from build123d import *

# Parameters (mm, degrees)
F0_R     = 10
F1_DEPTH = 5


with BuildPart() as f1:
    # F0 (on Front) → F1 (new body)
    with BuildSketch(Plane.XZ):
        Circle(F0_R)
        with BuildLine():
            ThreePointArc((-3.708099, -1.5), (-2.828427, -2.828427), (-1.5, -3.708099))
            Line((-1.5, -3.708099), (-1.5, -7.348469))
            ThreePointArc((-1.5, -7.348469), (-5.303301, -5.303301), (-7.348469, -1.5))
            Line((-7.348469, -1.5), (-3.708099, -1.5))
        make_face(mode=Mode.SUBTRACT)
        with BuildLine():
            Line((3.708099, -1.5), (7.348469, -1.5))
            ThreePointArc((7.348469, -1.5), (5.303301, -5.303301), (1.5, -7.348469))
            Line((1.5, -7.348469), (1.5, -3.708099))
            ThreePointArc((1.5, -3.708099), (2.828427, -2.828427), (3.708099, -1.5))
        make_face(mode=Mode.SUBTRACT)
        with BuildLine():
            Line((-1.5, 7.348469), (-1.5, 3.708099))
            ThreePointArc((-1.5, 3.708099), (-2.828427, 2.828427), (-3.708099, 1.5))
            Line((-3.708099, 1.5), (-7.348469, 1.5))
            ThreePointArc((-7.348469, 1.5), (-5.303301, 5.303301), (-1.5, 7.348469))
        make_face(mode=Mode.SUBTRACT)
        with BuildLine():
            Line((1.5, 3.708099), (1.5, 7.348469))
            ThreePointArc((1.5, 7.348469), (5.303301, 5.303301), (7.348469, 1.5))
            Line((7.348469, 1.5), (3.708099, 1.5))
            ThreePointArc((3.708099, 1.5), (2.828427, 2.828427), (1.5, 3.708099))
        make_face(mode=Mode.SUBTRACT)
    extrude(amount=F1_DEPTH)


solid = f1.part
Input: part model. Units: mm. Frame: model coordinates. A direction names the side the tool comes from. Round coordinates to 2 decimals unless told otherwise and drop trailing zeros. Order: outer loops, then holes, each group sorted by start corner. A loop starts at its lowest first (then second) coordinate and runs counter-clockwise, first axis right, second up.
1. Set-up query: faces 4 (the face through (0, -5, 0)), 5 (the face through (-6, -2, -1.5)). Return all of +Z, -Z, +X, -X, +Y, -Y with unobstructed straight access to the full face (end or side cutting, diameter ignored); none if empty.
The answers:
face 4: +Z, -Z, +X, -X, -Y
face 5: +Y, -Y
2. Cut plane A-A, the plane y = -4.05. Output: boundary loops of the cut face in (x, z).
The answers:
outline: circle Ø20 at (0, 0); hole (-7.35, -1.5) arc R7.5 ccw to (-1.5, -7.35) - (-1.5, -3.71) arc R4 cw to (-3.71, -1.5) - close; hole (-7.35, 1.5) - (-3.71, 1.5) arc R4 cw to (-1.5, 3.71) - (-1.5, 7.35) arc R7.5 ccw to start; hole (1.5, -7.35) arc R7.5 ccw to (7.35, -1.5) - (3.71, -1.5) arc R4 cw to (1.5, -3.71) - close; hole (1.5, 3.71) arc R4 cw to (3.71, 1.5) - (7.35, 1.5) arc R7.5 ccw to (1.5, 7.35) - close
3. Pin query (flat end, axial travel): P1, Ø1.8, axis at x = -5, y = -3.5, coming from the +Z side; P2, Ø10, axis at x = 2, z = -5, coming from the +Y side; P3, Ø3, axis at y = -2.5, z = -2.5, coming from the -X side; P4, Ø1.1, axis at x = 4.5, y = -3.5, coming from the -Z side. Return the tip coordinate at first contact, or that it passes through.
The answers:
P1: stops at z = 9.12
P2: stops at y = 0
P3: stops at x = -9.95
P4: stops at z = -9.19
4. Material intervals for line 1 (X direction, y = -1.65, z = -6); line 2 (Z direction, x = 2, y = -0.4); line 3 (Z direction, x = -4, y = -4.55), sorted ascending.
The answers:
line 1: x = -8 to -4.5, -1.5 to 1.5, 4.5 to 8
line 2: z = -9.8 to -7.23, -3.46 to 3.46, 7.23 to 9.8
line 3: z = -9.17 to -6.34, -1.5 to 1.5, 6.34 to 9.17
5. Mould query, pull axis Z, two halves, no side actions, for faces 1 (the face through (-2.17, -2.46, -9.76)), 2 (the face through (0, 0, 0)), 3 (the face through (2.844, -2.465, 2.813)). Classes: released by +Z, released by -Z, zero draft, split by the parting line, or undercut.
The answers:
face 1: split by the parting line
face 2: zero draft
face 3: undercut
